```python
from build123d import *

# Parameters (mm, degrees)
SKETCH1_R           = 25
SKETCH1_R_2         = 1.61
BOSS_EXTRUDE1_DEPTH = 7.5
CUT_EXTRUDE2_DEPTH  = 10


with BuildPart() as part:
    # Sketch1 → Boss-Extrude1 (new body)
    with BuildSketch(Plane(origin=(0, 0, 0), x_dir=(1, 0, 0), z_dir=(0, 1, 0))):
        Circle(SKETCH1_R)
        Circle(SKETCH1_R_2, mode=Mode.SUBTRACT)
    extrude(amount=BOSS_EXTRUDE1_DEPTH)

    # Sketch2 → Cut-Extrude2 (cut)
    with BuildSketch(Plane(origin=(0, 7.5, 0), x_dir=(1, 0, 0), z_dir=(0, 1, 0))):
        with BuildLine():
            Line((-1, 3.468731757), (-1, 22.978250586))
            ThreePointArc((-1, 22.978250586), (-13.519060803, 18.607390871), (-21.544597959, 8.051726448))
            Line((-21.544597959, 8.051726448), (-2.989942946, 2.022953578))
            ThreePointArc((-2.989942946, 2.022953578), (-2.121904761, 2.92055135), (-1, 3.468731757))
        make_face()
        with BuildLine():
            ThreePointArc((21.544597959, 8.051726448), (13.519060803, 18.607390871), (1, 22.978250586))
            Line((1, 22.978250586), (1, 3.468731757))
            ThreePointArc((1, 3.468731757), (2.121904761, 2.92055135), (2.989942946, 2.022953578))
            Line((2.989942946, 2.022953578), (21.544597959, 8.051726448))
        make_face()
        with BuildLine():
            ThreePointArc((23, 0), (22.789696518, 3.103181046), (22.162631947, 6.149613416))
            Line((22.162631947, 6.149613416), (3.607976935, 0.120840545))
            ThreePointArc((3.607976935, 0.120840545), (3.609494198, 0.060428739), (3.61, 0))
            ThreePointArc((3.61, 0), (3.41415947, -1.172866195), (2.847886365, -2.218477688))
            Line((2.847886365, -2.218477688), (14.315293812, -18.002009973))
            ThreePointArc((14.315293812, -18.002009973), (20.715353698, -9.993704076), (23, 0))
        make_face()
        with BuildLine():
            Line((-1.229852376, -3.394048192), (-12.697259824, -19.177580477))
            ThreePointArc((-12.697259824, -19.177580477), (0, -23), (12.697259824, -19.177580477))
            Line((12.697259824, -19.177580477), (1.229852376, -3.394048192))
            ThreePointArc((1.229852376, -3.394048192), (0, -3.61), (-1.229852376, -3.394048192))
        make_face()
        with BuildLine():
            Line((-3.607976935, 0.120840545), (-22.162631947, 6.149613416))
            ThreePointArc((-22.162631947, 6.149613416), (-21.874299875, -7.107390871), (-14.315293812, -18.002009973))
            Line((-14.315293812, -18.002009973), (-2.847886365, -2.218477688))
            ThreePointArc((-2.847886365, -2.218477688), (-3.433314024, -1.11555135), (-3.607976935, 0.120840545))
        make_face()
    extrude(amount=-CUT_EXTRUDE2_DEPTH, mode=Mode.SUBTRACT)


solid = part.part
```
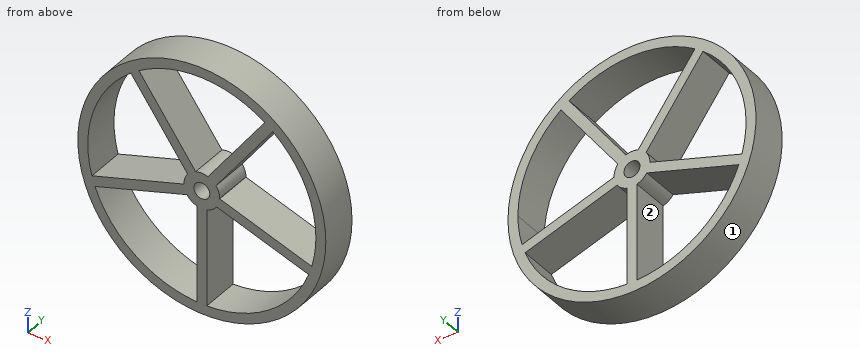
Part model, mm, in its own coordinate system. Face numbers are marked on the shaded views. Round coordinates to 2 decimals unless told otherwise and drop trailing zeros. Write each loop counter-clockwise with the first axis right and the second up, starting at its lowest first coordinate (ties: lowest second). Pieces come first, ordered by that corner, then holes. Notation, with made-up numbers: M -5.5,52 L 52.5,52 A21 ccw 52.5,81 Z; hole C -24.75,39 d3. An arc over 180 degrees is marked long. One line per question, with ' | ' between items.
(1) Probe line 1 along Z through (x, y) = (0, 2.5); line 2 along Z through (x, y) = (20, 4); line 3 along Z through (x, y) = (-9.5, 5.5). List the from-to ranges inside material, lowest first.
Answer key:
line 1: z = -25 to -1.61, 1.61 to 3.61, 23 to 25 | line 2: z = -15 to -11.36, -7.55 to -5.45, 11.36 to 15 | line 3: z = -23.12 to -20.95, -4.14 to -2.04, 11.37 to 14.78, 20.95 to 23.12
(2) Saw through at B-B on y = 4. Write the cut outline in (x, z).
Answer key:
outline: C 0,0 d50; hole M -22.16,-6.15 L -3.61,-0.12 A3.61 cw -2.85,2.22 L -14.32,18 A23 ccw Z; hole M -21.54,-8.05 A23 ccw -1,-22.98 L -1,-3.47 A3.61 cw -2.99,-2.02 Z; hole M -12.7,19.18 L -1.23,3.39 A3.61 cw 1.23,3.39 L 12.7,19.18 A23 ccw Z; hole C 0,0 d3.22; hole M 1,-22.98 A23 ccw 21.54,-8.05 L 2.99,-2.02 A3.61 cw 1,-3.47 Z; hole M 2.85,2.22 A3.61 cw 3.61,0 A3.61 cw 3.61,-0.12 L 22.16,-6.15 A23 ccw 14.32,18 Z
(3) Saw through at D-D on z = -7. Write the cut outline in (x, y), then the cut area to 3 significant figures.
Answer key:
outline: M -24,0 L -18.31,0 L -18.31,7.5 L -24,7.5 Z; M -1,0 L 1,0 L 1,7.5 L -1,7.5 Z; M 18.31,0 L 24,0 L 24,7.5 L 18.31,7.5 Z | area: 100 mm^2
(4) Pin check, flat tips, straight feed: pin 1 (1.5 mm diameter, centred on y = 6, z = -19.5, fed in from +X); pin 2 (1.5 mm diameter, centred on x = -12.5, y = 1, fed in from +Z); pin 3 (3 mm diameter, centred on y = 3, z = -5, fed in from -X); pin 4 (1.9 mm diameter, centred on x = 0, z = 0, fed in from -Y). Stop position of each tip, or through.
Answer key:
pin 1: stops at x = 16.54 | pin 2: stops at z = 22.07 | pin 3: stops at x = -24.75 | pin 4: passes through
(5) Saw through at C-C on z = 10.5. Write the cut outline in (x, y), then the cut area to 3 significant figures.
Answer key:
outline: M -22.69,0 L -20.46,0 L -20.46,7.5 L -22.69,7.5 Z; M -8.86,0 L -6.39,0 L -6.39,7.5 L -8.86,7.5 Z; M 6.39,0 L 8.86,0 L 8.86,7.5 L 6.39,7.5 Z; M 20.46,0 L 22.69,0 L 22.69,7.5 L 20.46,7.5 Z | area: 70.5 mm^2
(6) Two-plate mould, pull along X, no slides. Class the marked faces 1 and 2: released by +X, released by -X, zero draft, split by the parting line, or undercut.
Answer key:
face 1: split by the parting line | face 2: undercut
(7) Saw through at A-A on x = 0. Write the cut outline in (y, z), then the cut area to 3 significant figures.
Answer key:
outline: M 0,-25 L 7.5,-25 L 7.5,-1.61 L 0,-1.61 Z; M 0,1.61 L 7.5,1.61 L 7.5,3.61 L 0,3.61 Z; M 0,23 L 7.5,23 L 7.5,25 L 0,25 Z | area: 205 mm^2
